```python
from build123d import *

# Parameters (mm, degrees)
SKETCH_1_W      = 2.5
SKETCH_1_H      = 7.5
EXTRUDE_1_DEPTH = 5
SKETCH_2_W      = 2
SKETCH_2_H      = 2
EXTRUDE_2_DEPTH = 3
SKETCH_3_R      = 0.5


with BuildPart() as part:
    # 草图1 → 凸台-拉伸1 (new body)
    with BuildSketch(Plane.XY):
        with Locations((1.25, -10.035009445)):
            Rectangle(SKETCH_1_W, SKETCH_1_H)
    extrude(amount=EXTRUDE_1_DEPTH)

    # 草图2 → 凸台-拉伸2 (add)
    with BuildSketch(Plane(origin=(2.5, 0, 0), x_dir=(0, 0, -1), z_dir=(1, 0, 0))):
        with Locations((-2.5, -7.530464336)):
            Rectangle(SKETCH_2_W, SKETCH_2_H)
    extrude(amount=EXTRUDE_2_DEPTH)

    # 扫描1: sweep along a path in 草图4
    with BuildLine(Plane.XZ.offset(10.035009445)) as sweep_1_path:
        Line((0, 3.097044355), (-2, 3.097044355))
        Line((-2, 3.097044355), (-2, -2))
    # 草图3 → 扫描1 (sweep)
    with BuildSketch(Plane.ZY):
        with Locations((2.592115007, -10.035009445)):
            Circle(SKETCH_3_R)
        with Locations((2.592115007, -7.495009445)):
            Circle(SKETCH_3_R)
        with Locations((2.592115007, -12.575009445)):
            Circle(SKETCH_3_R)
    sweep(path=sweep_1_path.line, transition=Transition.RIGHT)


solid = part.part
```
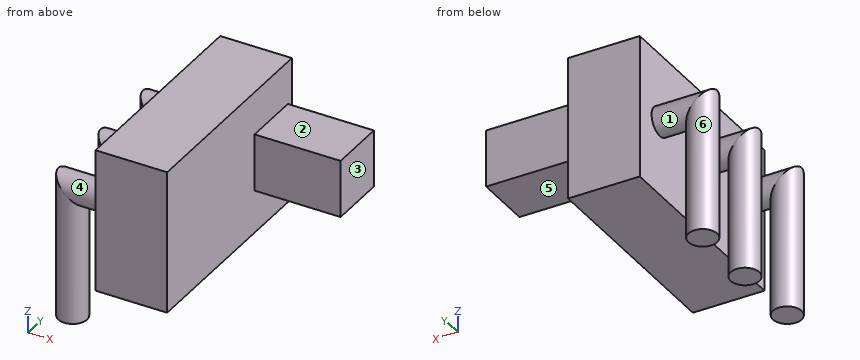
Verification items for the finished model (mm, model axes). Face numbers are marked on the shaded views. A direction names the side the tool comes from. Coordinates: 2 decimals unless noted, no trailing zeros. Write each loop counter-clockwise with the first axis right and the second up, starting at its lowest first coordinate (ties: lowest second). Pieces come first, ordered by that corner, then holes. Notation, with made-up numbers: (-22, 24.5) - (6, 24.5) arc R23 cw to (6, 53.5) - close; hole circle Ø2 at (-13, -30). An arc over 180 degrees is marked (long way). Write item = value, one per line.
Q1. Cross-section at C-C (x = 5). Enter the section's corners in (y, z).
Answer:
outline = (-8.53, 1.5) - (-6.53, 1.5) - (-6.53, 3.5) - (-8.53, 3.5) - close
Q2. Access from +Z, -Z, +X, -X, +Y, -Y to the whole of each face (thin tool, end or side, straight path). Record for the marked faces 4, 5 and 6.
Answer:
face_4 = none
face_5 = -Z, +X, +Y, -Y
face_6 = -Z
Q3. Go/stop test with flat-tipped pins: pin 1 Ø1.6 at (x, z) = (4, 3) entering from +Y; pin 2 Ø0.6 at (x, y) = (4, -7.5) entering from +Z; pin 3 Ø1 at (x, z) = (3.5, 2.5) entering from -Y. Record where each tip stops, or that it passes through.
Answer:
pin_1 = -6.53
pin_2 = 3.5
pin_3 = -8.53
Q4. Cross-section at A-A (z = 1.25). Enter the section's corners in (x, y) (3 decimals).
Answer:
outline = circle Ø1 at (-1.495, -12.575); circle Ø1 at (-1.495, -10.035); circle Ø1 at (-1.495, -7.495); (0, -13.785) - (2.5, -13.785) - (2.5, -6.285) - (0, -6.285) - close
Q5. Cross-section at B-B (y = -8.25). Enter the section's corners in (x, z).
Answer:
outline = (0, 0) - (2.5, 0) - (2.5, 1.5) - (5.5, 1.5) - (5.5, 3.5) - (2.5, 3.5) - (2.5, 5) - (0, 5) - close
Q6. Cross-section at D-D (x = -0.25). Enter the section's corners in (y, z) (3 decimals), plus the area to 3 significant figures.
Answer:
outline = circle Ø1 at (-12.575, 2.592); circle Ø1 at (-10.035, 2.592); circle Ø1 at (-7.495, 2.592)
area = 2.36 mm²
Q7. Mould release check, pull along X, two halves, no side actions. Record for the marked faces 1, 2 and 3: released by +X, released by -X, zero draft, split by the parting line, or undercut.
Answer:
face_1 = undercut
face_2 = zero draft
face_3 = released by +X
Q8. Material ranges on L1, parallel to Y at x = -0.5, z = 2.75; L2, parallel to X at y = -9.5, z = 1.5; L3, parallel to Z at x = 4.75, y = -8.5, recorded low to high. Write a range as from..to.
Answer:
L1 = -13.05..-12.1, -10.51..-9.56, -7.97..-7.02
L2 = 0..2.5
L3 = 1.5..3.5
